Verification items for the finished model (mm, model axes). Face numbers are marked on the shaded views. Round coordinates to 2 decimals unless told otherwise and drop trailing zeros. Order: outer loops, then holes, each group sorted by start corner. A loop starts at its lowest first (then second) coordinate and runs counter-clockwise, first axis right, second up. Notation, with made-up numbers: (-1, 17) -> (42, 17) arc R19 ccw to (42, 35) -> close; hole circle Ø11 at (51, 52). An arc over 180 degrees is marked (long way). Return JSON: item names as keys, results as strings. Group by question number.
Item 1: Depth check by flat-ended pin: pin 1 Ø10 at (x, y) = (27, 20.5) entering from -Z. Enter the tip coordinate at first touch or a pass-through.
Item 2: Sectioned sample at A-A on y = 14.5. Record the cut outline in (x, z).
Item 3: Draft check along Y on the marked faces 1, 2 and 3. Enter one of: pulls with the +Y half, pulls with the -Y half, needs draft (parallel to the pull), parting line crosses it, or undercut.
Item 4: Scan lines: probe 1 along Z at (x, y) = (44.5, 16); probe 2 along Y at (x, z) = (63.5, -0.25); probe 3 along X at (y, z) = (4.5, 3.25). Record each from-to range of solid material in increasing order. Write a range as from..to.
```python
from build123d import *

# Parameters (mm, degrees)
ESQUISSE1_W                     = 85
ESQUISSE1_H                     = 40
BOSS_EXTRU_1_DEPTH              = 6
CONG_1_R                        = 5
ESQUISSE2_R                     = 4.5
BOSS_EXTRU_2_DEPTH              = 1
R_P_TITION_LIN_AIRE1_COUNT      = 7
R_P_TITION_LIN_AIRE1_PITCH      = 11
R_P_TITION_LIN_AIRE1_COUNT_DIR2 = 3
R_P_TITION_LIN_AIRE1_PITCH_DIR2 = 11
CONG_2_R                        = 5


with BuildPart() as part:
    # Esquisse1 → Boss.-Extru.1 (new body)
    with BuildSketch(Plane.XY):
        with Locations((42.5, 20)):
            Rectangle(ESQUISSE1_W, ESQUISSE1_H)
    extrude(amount=BOSS_EXTRU_1_DEPTH)

    # Congé1
    cong_1_edges = [part.edges().sort_by_distance(p)[0] for p in [
        (0, 40, 3),
        (85, 40, 3),
        (85, 0, 3),
        (0, 0, 3),
    ]]
    fillet(cong_1_edges, radius=CONG_1_R)

    # Esquisse2 → Boss.-Extru.2 (add)
    with BuildSketch(Plane(origin=(0, 0, 0), x_dir=(-1, 0, 0), z_dir=(0, 0, -1))):
        with Locations((-9, 31)):
            Circle(ESQUISSE2_R)
    boss_extru_2 = extrude(amount=BOSS_EXTRU_2_DEPTH)

    # Répétition linéaire1: Boss.-Extru.2 7 × 3
    with Locations(*[(i * R_P_TITION_LIN_AIRE1_PITCH, -j * R_P_TITION_LIN_AIRE1_PITCH_DIR2, 0) for i in range(R_P_TITION_LIN_AIRE1_COUNT) for j in range(R_P_TITION_LIN_AIRE1_COUNT_DIR2) if (i, j) != (0, 0)]):
        add(boss_extru_2)

    # Congé2
    # the kernel refuses this fillet: 5 mm, written as the material it takes off along each edge
    with BuildSketch(Plane(origin=(9, 31, -1), x_dir=(-1, 0, 0), z_dir=(0, -1, 0))) as cong_2_piece_1:
        with BuildLine():
            CenterArc((1.5, -5), CONG_2_R, 53.130102354, 36.869897646)
            Line((1.5, 0), (1.5, 0.1))
            Line((1.5, 0.1), (4.5, 0.1))
            Line((4.5, 0.1), (4.6, 0))
            ThreePointArc((4.6, 0), (4.6, -0.5), (4.56, -0.92))
            Line((4.56, -0.92), (4.5, -1))
        make_face()
    revolve(axis=Axis((9, 31, -1), (0, 0, -1)), mode=Mode.SUBTRACT)
    with BuildSketch(Plane(origin=(20, 20, -1), x_dir=(-1, 0, 0), z_dir=(0, -1, 0))) as cong_2_piece_2:
        with BuildLine():
            CenterArc((1.5, -5), CONG_2_R, 53.130102354, 36.869897646)
            Line((1.5, 0), (1.5, 0.1))
            Line((1.5, 0.1), (4.5, 0.1))
            Line((4.5, 0.1), (4.6, 0))
            ThreePointArc((4.6, 0), (4.6, -0.5), (4.56, -0.92))
            Line((4.56, -0.92), (4.5, -1))
        make_face()
    revolve(axis=Axis((20, 20, -1), (0, 0, -1)), mode=Mode.SUBTRACT)
    with BuildSketch(Plane(origin=(31, 20, -1), x_dir=(-1, 0, 0), z_dir=(0, -1, 0))) as cong_2_piece_3:
        with BuildLine():
            CenterArc((1.5, -5), CONG_2_R, 53.130102354, 36.869897646)
            Line((1.5, 0), (1.5, 0.1))
            Line((1.5, 0.1), (4.5, 0.1))
            Line((4.5, 0.1), (4.6, 0))
            ThreePointArc((4.6, 0), (4.6, -0.5), (4.56, -0.92))
            Line((4.56, -0.92), (4.5, -1))
        make_face()
    revolve(axis=Axis((31, 20, -1), (0, 0, -1)), mode=Mode.SUBTRACT)
    with BuildSketch(Plane(origin=(42, 20, -1), x_dir=(-1, 0, 0), z_dir=(0, -1, 0))) as cong_2_piece_4:
        with BuildLine():
            CenterArc((1.5, -5), CONG_2_R, 53.130102354, 36.869897646)
            Line((1.5, 0), (1.5, 0.1))
            Line((1.5, 0.1), (4.5, 0.1))
            Line((4.5, 0.1), (4.6, 0))
            ThreePointArc((4.6, 0), (4.6, -0.5), (4.56, -0.92))
            Line((4.56, -0.92), (4.5, -1))
        make_face()
    revolve(axis=Axis((42, 20, -1), (0, 0, -1)), mode=Mode.SUBTRACT)
    with BuildSketch(Plane(origin=(53, 20, -1), x_dir=(-1, 0, 0), z_dir=(0, -1, 0))) as cong_2_piece_5:
        with BuildLine():
            CenterArc((1.5, -5), CONG_2_R, 53.130102354, 36.869897646)
            Line((1.5, 0), (1.5, 0.1))
            Line((1.5, 0.1), (4.5, 0.1))
            Line((4.5, 0.1), (4.6, 0))
            ThreePointArc((4.6, 0), (4.6, -0.5), (4.56, -0.92))
            Line((4.56, -0.92), (4.5, -1))
        make_face()
    revolve(axis=Axis((53, 20, -1), (0, 0, -1)), mode=Mode.SUBTRACT)
    with BuildSketch(Plane(origin=(64, 20, -1), x_dir=(-1, 0, 0), z_dir=(0, -1, 0))) as cong_2_piece_6:
        with BuildLine():
            CenterArc((1.5, -5), CONG_2_R, 53.130102354, 36.869897646)
            Line((1.5, 0), (1.5, 0.1))
            Line((1.5, 0.1), (4.5, 0.1))
            Line((4.5, 0.1), (4.6, 0))
            ThreePointArc((4.6, 0), (4.6, -0.5), (4.56, -0.92))
            Line((4.56, -0.92), (4.5, -1))
        make_face()
    revolve(axis=Axis((64, 20, -1), (0, 0, -1)), mode=Mode.SUBTRACT)
    with BuildSketch(Plane(origin=(9, 20, -1), x_dir=(-1, 0, 0), z_dir=(0, -1, 0))) as cong_2_piece_7:
        with BuildLine():
            CenterArc((1.5, -5), CONG_2_R, 53.130102354, 36.869897646)
            Line((1.5, 0), (1.5, 0.1))
            Line((1.5, 0.1), (4.5, 0.1))
            Line((4.5, 0.1), (4.6, 0))
            ThreePointArc((4.6, 0), (4.6, -0.5), (4.56, -0.92))
            Line((4.56, -0.92), (4.5, -1))
        make_face()
    revolve(axis=Axis((9, 20, -1), (0, 0, -1)), mode=Mode.SUBTRACT)
    with BuildSketch(Plane(origin=(9, 9, -1), x_dir=(-1, 0, 0), z_dir=(0, -1, 0))) as cong_2_piece_8:
        with BuildLine():
            CenterArc((1.5, -5), CONG_2_R, 53.130102354, 36.869897646)
            Line((1.5, 0), (1.5, 0.1))
            Line((1.5, 0.1), (4.5, 0.1))
            Line((4.5, 0.1), (4.6, 0))
            ThreePointArc((4.6, 0), (4.6, -0.5), (4.56, -0.92))
            Line((4.56, -0.92), (4.5, -1))
        make_face()
    revolve(axis=Axis((9, 9, -1), (0, 0, -1)), mode=Mode.SUBTRACT)
    with BuildSketch(Plane(origin=(20, 31, -1), x_dir=(-1, 0, 0), z_dir=(0, -1, 0))) as cong_2_piece_9:
        with BuildLine():
            CenterArc((1.5, -5), CONG_2_R, 53.130102354, 36.869897646)
            Line((1.5, 0), (1.5, 0.1))
            Line((1.5, 0.1), (4.5, 0.1))
            Line((4.5, 0.1), (4.6, 0))
            ThreePointArc((4.6, 0), (4.6, -0.5), (4.56, -0.92))
            Line((4.56, -0.92), (4.5, -1))
        make_face()
    revolve(axis=Axis((20, 31, -1), (0, 0, -1)), mode=Mode.SUBTRACT)
    with BuildSketch(Plane(origin=(20, 9, -1), x_dir=(-1, 0, 0), z_dir=(0, -1, 0))) as cong_2_piece_10:
        with BuildLine():
            CenterArc((1.5, -5), CONG_2_R, 53.130102354, 36.869897646)
            Line((1.5, 0), (1.5, 0.1))
            Line((1.5, 0.1), (4.5, 0.1))
            Line((4.5, 0.1), (4.6, 0))
            ThreePointArc((4.6, 0), (4.6, -0.5), (4.56, -0.92))
            Line((4.56, -0.92), (4.5, -1))
        make_face()
    revolve(axis=Axis((20, 9, -1), (0, 0, -1)), mode=Mode.SUBTRACT)
    with BuildSketch(Plane(origin=(31, 31, -1), x_dir=(-1, 0, 0), z_dir=(0, -1, 0))) as cong_2_piece_11:
        with BuildLine():
            CenterArc((1.5, -5), CONG_2_R, 53.130102354, 36.869897646)
            Line((1.5, 0), (1.5, 0.1))
            Line((1.5, 0.1), (4.5, 0.1))
            Line((4.5, 0.1), (4.6, 0))
            ThreePointArc((4.6, 0), (4.6, -0.5), (4.56, -0.92))
            Line((4.56, -0.92), (4.5, -1))
        make_face()
    revolve(axis=Axis((31, 31, -1), (0, 0, -1)), mode=Mode.SUBTRACT)
    with BuildSketch(Plane(origin=(31, 9, -1), x_dir=(-1, 0, 0), z_dir=(0, -1, 0))) as cong_2_piece_12:
        with BuildLine():
            CenterArc((1.5, -5), CONG_2_R, 53.130102354, 36.869897646)
            Line((1.5, 0), (1.5, 0.1))
            Line((1.5, 0.1), (4.5, 0.1))
            Line((4.5, 0.1), (4.6, 0))
            ThreePointArc((4.6, 0), (4.6, -0.5), (4.56, -0.92))
            Line((4.56, -0.92), (4.5, -1))
        make_face()
    revolve(axis=Axis((31, 9, -1), (0, 0, -1)), mode=Mode.SUBTRACT)
    with BuildSketch(Plane(origin=(42, 31, -1), x_dir=(-1, 0, 0), z_dir=(0, -1, 0))) as cong_2_piece_13:
        with BuildLine():
            CenterArc((1.5, -5), CONG_2_R, 53.130102354, 36.869897646)
            Line((1.5, 0), (1.5, 0.1))
            Line((1.5, 0.1), (4.5, 0.1))
            Line((4.5, 0.1), (4.6, 0))
            ThreePointArc((4.6, 0), (4.6, -0.5), (4.56, -0.92))
            Line((4.56, -0.92), (4.5, -1))
        make_face()
    revolve(axis=Axis((42, 31, -1), (0, 0, -1)), mode=Mode.SUBTRACT)
    with BuildSketch(Plane(origin=(42, 9, -1), x_dir=(-1, 0, 0), z_dir=(0, -1, 0))) as cong_2_piece_14:
        with BuildLine():
            CenterArc((1.5, -5), CONG_2_R, 53.130102354, 36.869897646)
            Line((1.5, 0), (1.5, 0.1))
            Line((1.5, 0.1), (4.5, 0.1))
            Line((4.5, 0.1), (4.6, 0))
            ThreePointArc((4.6, 0), (4.6, -0.5), (4.56, -0.92))
            Line((4.56, -0.92), (4.5, -1))
        make_face()
    revolve(axis=Axis((42, 9, -1), (0, 0, -1)), mode=Mode.SUBTRACT)
    with BuildSketch(Plane(origin=(53, 31, -1), x_dir=(-1, 0, 0), z_dir=(0, -1, 0))) as cong_2_piece_15:
        with BuildLine():
            CenterArc((1.5, -5), CONG_2_R, 53.130102354, 36.869897646)
            Line((1.5, 0), (1.5, 0.1))
            Line((1.5, 0.1), (4.5, 0.1))
            Line((4.5, 0.1), (4.6, 0))
            ThreePointArc((4.6, 0), (4.6, -0.5), (4.56, -0.92))
            Line((4.56, -0.92), (4.5, -1))
        make_face()
    revolve(axis=Axis((53, 31, -1), (0, 0, -1)), mode=Mode.SUBTRACT)
    with BuildSketch(Plane(origin=(53, 9, -1), x_dir=(-1, 0, 0), z_dir=(0, -1, 0))) as cong_2_piece_16:
        with BuildLine():
            CenterArc((1.5, -5), CONG_2_R, 53.130102354, 36.869897646)
            Line((1.5, 0), (1.5, 0.1))
            Line((1.5, 0.1), (4.5, 0.1))
            Line((4.5, 0.1), (4.6, 0))
            ThreePointArc((4.6, 0), (4.6, -0.5), (4.56, -0.92))
            Line((4.56, -0.92), (4.5, -1))
        make_face()
    revolve(axis=Axis((53, 9, -1), (0, 0, -1)), mode=Mode.SUBTRACT)
    with BuildSketch(Plane(origin=(64, 31, -1), x_dir=(-1, 0, 0), z_dir=(0, -1, 0))) as cong_2_piece_17:
        with BuildLine():
            CenterArc((1.5, -5), CONG_2_R, 53.130102354, 36.869897646)
            Line((1.5, 0), (1.5, 0.1))
            Line((1.5, 0.1), (4.5, 0.1))
            Line((4.5, 0.1), (4.6, 0))
            ThreePointArc((4.6, 0), (4.6, -0.5), (4.56, -0.92))
            Line((4.56, -0.92), (4.5, -1))
        make_face()
    revolve(axis=Axis((64, 31, -1), (0, 0, -1)), mode=Mode.SUBTRACT)
    with BuildSketch(Plane(origin=(64, 9, -1), x_dir=(-1, 0, 0), z_dir=(0, -1, 0))) as cong_2_piece_18:
        with BuildLine():
            CenterArc((1.5, -5), CONG_2_R, 53.130102354, 36.869897646)
            Line((1.5, 0), (1.5, 0.1))
            Line((1.5, 0.1), (4.5, 0.1))
            Line((4.5, 0.1), (4.6, 0))
            ThreePointArc((4.6, 0), (4.6, -0.5), (4.56, -0.92))
            Line((4.56, -0.92), (4.5, -1))
        make_face()
    revolve(axis=Axis((64, 9, -1), (0, 0, -1)), mode=Mode.SUBTRACT)
    with BuildSketch(Plane(origin=(75, 31, -1), x_dir=(-1, 0, 0), z_dir=(0, -1, 0))) as cong_2_piece_19:
        with BuildLine():
            CenterArc((1.5, -5), CONG_2_R, 53.130102354, 36.869897646)
            Line((1.5, 0), (1.5, 0.1))
            Line((1.5, 0.1), (4.5, 0.1))
            Line((4.5, 0.1), (4.6, 0))
            ThreePointArc((4.6, 0), (4.6, -0.5), (4.56, -0.92))
            Line((4.56, -0.92), (4.5, -1))
        make_face()
    revolve(axis=Axis((75, 31, -1), (0, 0, -1)), mode=Mode.SUBTRACT)
    with BuildSketch(Plane(origin=(75, 20, -1), x_dir=(-1, 0, 0), z_dir=(0, -1, 0))) as cong_2_piece_20:
        with BuildLine():
            CenterArc((1.5, -5), CONG_2_R, 53.130102354, 36.869897646)
            Line((1.5, 0), (1.5, 0.1))
            Line((1.5, 0.1), (4.5, 0.1))
            Line((4.5, 0.1), (4.6, 0))
            ThreePointArc((4.6, 0), (4.6, -0.5), (4.56, -0.92))
            Line((4.56, -0.92), (4.5, -1))
        make_face()
    revolve(axis=Axis((75, 20, -1), (0, 0, -1)), mode=Mode.SUBTRACT)
    with BuildSketch(Plane(origin=(75, 9, -1), x_dir=(-1, 0, 0), z_dir=(0, -1, 0))) as cong_2_piece_21:
        with BuildLine():
            CenterArc((1.5, -5), CONG_2_R, 53.130102354, 36.869897646)
            Line((1.5, 0), (1.5, 0.1))
            Line((1.5, 0.1), (4.5, 0.1))
            Line((4.5, 0.1), (4.6, 0))
            ThreePointArc((4.6, 0), (4.6, -0.5), (4.56, -0.92))
            Line((4.56, -0.92), (4.5, -1))
        make_face()
    revolve(axis=Axis((75, 9, -1), (0, 0, -1)), mode=Mode.SUBTRACT)


solid = part.part
```
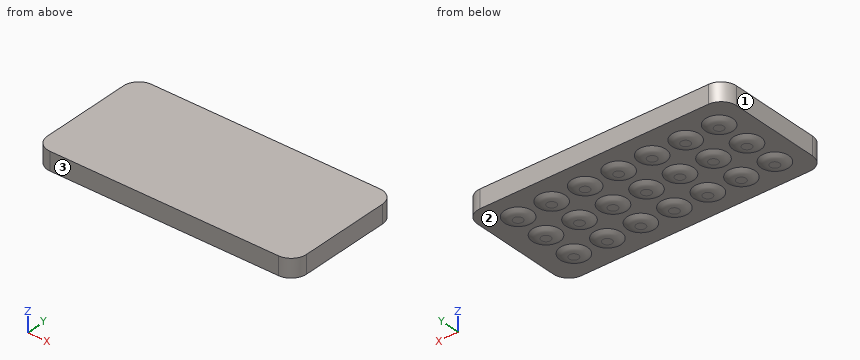
Recorded:
{
 "1": {"pin 1": "z = -1"},
 "2": {"outline": "(0, 0) -> (85, 0) -> (85, 6) -> (0, 6) -> close"},
 "3": {"face 1": "needs draft", "face 2": "undercut", "face 3": "pulls with the -Y half"},
 "4": {"probe 1": "0..6", "probe 2": "4.9..13.1, 15.9..24.1, 26.9..35.1", "probe 3": "0.03..84.97"}
}
